The listing builds one solid part. Answer for the finished solid, in the listing's coordinates (mm). Face numbers are marked on the shaded views. Coordinates: 2 decimals unless noted, no trailing zeros. Loops run counter-clockwise (first coordinate to the right, second up) from the corner with the lowest first, then second, coordinate; pieces in that order, holes last. Notation, with made-up numbers: M -37.75,62.5 L -19.75,62.5 A24 ccw -19.75,82.5 Z; hole C -24.75,63.5 d8. An arc over 180 degrees is marked long. Return JSON: item names as keys, results as strings. Group by question number.
1. Straight lines are drawn through the part: L1, parallel to Z at x = 1, y = 0; L2, parallel to Y at x = 0.95, z = -5; L3, parallel to Z at x = 1.05, y = -1.25. For each, find the intervals that lie inside material, in ascending order. Write a range as from..to.
2. Section A-A (z = -5) is taken. Write down the section's boundary in (x, y).
3. Given P1, Ø1.8, axis at y = 0, z = -5, coming from the +X side, flat-ended and moving along its own axis, determine where the tip first touches the part or whether it passes through.
4. Section C-C (x = 0.6) is taken. Write down the section's boundary in (y, z), then the cut area to 3 significant figures.
5. Section D-D (z = 3.75) is taken. Write down the section's boundary in (x, y).
6. The mould has two halves that part along Z. Classify the marked faces 1 and 2: pulls with the +Z half, pulls with the -Z half, needs draft (parallel to the pull), parting line crosses it, or undercut.
7. Section B-B (y = 0) is taken. Write down the section's boundary in (x, z), then the cut area to 3 significant figures.
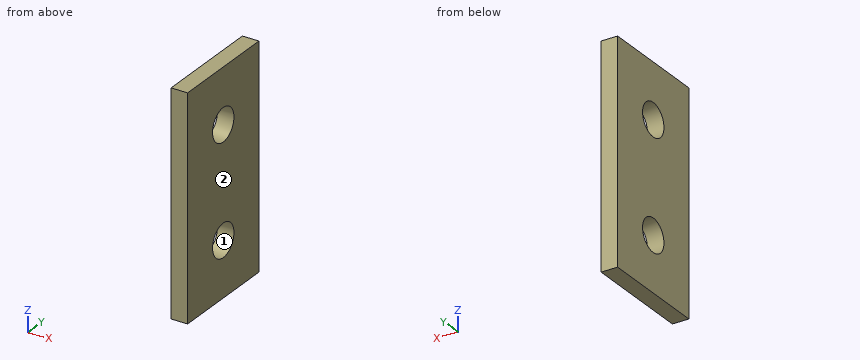
Autodesk Inventor part; units mm, degrees
ref_plane "YZ Plane" through (0, 0, 0) normal (1, 0, 0) x (0, 1, 0)
ref_plane "XZ Plane" through (0, 0, 0) normal (0, 1, 0) x (-1, 0, 0)
ref_plane "XY Plane" through (0, 0, 0) normal (0, 0, 1) x (1, 0, 0)
sketch "Sketch1" plane through (0, 0, 0) normal (1, 0, 0) x (0, 1, 0)
  line L0 (5, 10) -> (-5, 10)
  line L1 (-5, 10) -> (-5, -10)
  line L2 (-5, -10) -> (5, -10)
  line L3 (5, -10) -> (5, 10)
  line L4 (5, 10) -> (-5, -10) construction
  line L5 (-5, 10) -> (5, -10) construction
  line L6 (0, 0) -> (0, -5)
  line L7 (0, -5) -> (0, 5)
  circle A0 centre (0, 5) radius 1.5
  circle A1 centre (0, -5) radius 1.5
  dimension "d0" = 10
  dimension "d1" = 20
  dimension "d2" = 5
  dimension "d3" = 10
  dimension "d4" = 3
  dimension "d5" = 3
extrude "Extrusion1" add sketch "Sketch1" along normal blind 1.5
properties part number "kundi"
Worked out:
{
 "1": {"L1": "-10..-6.5, -3.5..3.5, 6.5..10", "L2": "-5..-1.5, 1.5..5", "L3": "-10..-5.83, -4.17..4.17, 5.83..10"},
 "2": {"outline": "M 0,-5 L 1.5,-5 L 1.5,-1.5 L 0,-1.5 Z; M 0,1.5 L 1.5,1.5 L 1.5,5 L 0,5 Z"},
 "3": {"P1": "through"},
 "4": {"outline": "M -5,-10 L 5,-10 L 5,10 L -5,10 Z; hole C 0,-5 d3; hole C 0,5 d3", "area": "186 mm^2"},
 "5": {"outline": "M 0,-5 L 1.5,-5 L 1.5,-0.83 L 0,-0.83 Z; M 0,0.83 L 1.5,0.83 L 1.5,5 L 0,5 Z"},
 "6": {"face 1": "undercut", "face 2": "needs draft"},
 "7": {"outline": "M 0,-10 L 1.5,-10 L 1.5,-6.5 L 0,-6.5 Z; M 0,-3.5 L 1.5,-3.5 L 1.5,3.5 L 0,3.5 Z; M 0,6.5 L 1.5,6.5 L 1.5,10 L 0,10 Z", "area": "21.0 mm^2"}
}
